Could you check a few things on this model? Use its own coordinates, in mm. Coordinates: 2 decimals unless noted, no trailing zeros. Loops run counter-clockwise (first coordinate to the right, second up) from the corner with the lowest first, then second, coordinate; pieces in that order, holes last.
1) Will these pins go through, and if not, where does the flat tip stop? P1, Ø10, axis at x = 28.5, z = 27.5, coming from the -Y side; P2, Ø1.5, axis at y = 19, z = -15.5, coming from the -X side; P3, Ø6, axis at x = -24.5, y = 19.5, coming from the -Z side; P4, Ø1, axis at x = 33, y = 13, coming from the -Z side.
2) Thinking about a two-plate mould opening in Z: for faces 1 (the face through (-30.911, 11.646, -40.313)), 2 (the face through (-49, 23.622, 11)), 3 (the face through (48.684, 11.886, -12.022)), which applies, released by +Z, released by -Z, zero draft, split by the parting line, or undercut?
3) If I drill on line 1 along X through (y, z) = (11.25, 0); line 2 along Z through (x, y) = (19, 19.75); line 3 along X through (y, z) = (17.25, -2.5), over which ranges is the centre line in solid material (lowest first)?
4) Imagine slicing it at C-C on y = 21. Please give me the cut outline in (x, z).
5) Imagine slicing it at A-A on z = 0. Please give me the cut outline in (x, y), plus the area to 3 significant figures.
6) Imagine slicing it at B-B on x = -5.5. Please give me the cut outline in (y, z).
```python
from build123d import *

# Parameters (mm, degrees)
SKETCH1_R           = 50.8
SKETCH1_R_2         = 49.53
BOSS_EXTRUDE1_DEPTH = 23.622
SKETCH2_R           = 2.38125
CUT_EXTRUDE1_DEPTH  = 25.4
SKETCH3_R           = 1.5875
CUT_EXTRUDE2_DEPTH  = 37.338
CIRPATTERN1_COUNT   = 4


with BuildPart() as part:
    # Sketch1 → Boss-Extrude1 (new body)
    with BuildSketch(Plane(origin=(0, 0, 0), x_dir=(1, 0, 0), z_dir=(0, 1, 0))):
        with Locations(Location((0, 0, 0), (0, 0, 270))):
            Circle(SKETCH1_R)
        with Locations(Location((0, 0, 0), (0, 0, 270))):
            Circle(SKETCH1_R_2, mode=Mode.SUBTRACT)
    extrude(amount=BOSS_EXTRUDE1_DEPTH)

    # Sketch2 → Cut-Extrude1 (cut)
    with BuildSketch(Plane(origin=(80.709285485, 206.333156205, 111.645979585), x_dir=(0, -1, 0), z_dir=(0.9693386284605577, 0, -0.2457287597620699))):
        with Locations(Location((196.808156205, 128.055353348, 0), (0, 0, 90))):
            Circle(SKETCH2_R)
        with Locations(Location((190.458156205, 128.055353348, 0), (0, 0, 90))):
            Circle(SKETCH2_R)
    extrude(amount=-CUT_EXTRUDE1_DEPTH, mode=Mode.SUBTRACT)

    # Sketch3 → Cut-Extrude2 (cut)
    with BuildSketch(Plane(origin=(-3.10026152, 207.778194099, 134.798971935), x_dir=(0, 1, 0), z_dir=(-0.962336256997443, 0, -0.27186196583588446))):
        with Locations(Location((-195.078194099, 130.56478129, 0), (0, 0, 270))):
            Circle(SKETCH3_R)
    cut_extrude2 = extrude(amount=-CUT_EXTRUDE2_DEPTH, mode=Mode.SUBTRACT)

    # CirPattern1: Cut-Extrude2 ×4 about axis
    cirpattern1_axis = Axis((0, 0, 0), (0, -1, 0))
    for i in range(1, CIRPATTERN1_COUNT):
        add(cut_extrude2.rotate(cirpattern1_axis, i * 360 / CIRPATTERN1_COUNT), mode=Mode.SUBTRACT)


solid = part.part
```
Filled in:
1. P1: passes through
1. P2: stops at x = -48.61
1. P3: stops at z = -46.03
1. P4: stops at z = -39.04
2. face 1: split by the parting line
2. face 2: zero draft
2. face 3: undercut
3. line 1: x = -50.8 to -49.53, 49.53 to 50.8
3. line 2: z = -47.11 to -45.74, 45.74 to 47.11
3. line 3: x = -50.74 to -49.47, 49.47 to 50.74
4. outline: circle Ø101.6 at (0, 0); hole circle Ø99.06 at (0, 0)
5. outline: (-50.8, 0) - (-49.53, 0) - (-49.53, 23.62) - (-50.8, 23.62) - close; (49.53, 0) - (50.8, 0) - (50.8, 23.62) - (49.53, 23.62) - close
5. area: 60.0 mm2
6. outline: (0, -50.5) - (23.62, -50.5) - (23.62, -49.22) - (0, -49.22) - close; (0, 49.22) - (23.62, 49.22) - (23.62, 50.5) - (0, 50.5) - close
